```python
from build123d import *

# Parameters (mm, degrees)
ESQUISSE1_R             = 1.6
BOSS_EXTRU_1_DEPTH      = 3
BOSS_EXTRU_2_START      = 4
ESQUISSE2_R             = 2.734743529
ESQUISSE2_R_2           = 1.6
BOSS_EXTRU_2_DEPTH      = 4
ENL_V_MAT_EXTRU_1_DEPTH = 3


with BuildPart() as part:
    # Esquisse1 → Boss.-Extru.1 (new body)
    with BuildSketch(Plane(origin=(0, 0, 0), x_dir=(1, 0, 0), z_dir=(0, 1, 0))):
        with BuildLine():
            Line((-19, 3), (19, 3))
            add(Edge.make_bspline(
                [(19, 3), (20.68639149, 3.094620003), (23.315621509, 0.000753175), (20.682364624, -3.097569459), (19, -3)],
                knots=[0, 0, 0, 0, 0.499941737, 1, 1, 1, 1], degree=3))
            Line((19, -3), (-19, -3))
            add(Edge.make_bspline(
                [(-19, 3), (-20.661097815, 3.102497637), (-23.341647105, 0.00157467), (-20.655607875, -3.105760191), (-19, -3)],
                knots=[0, 0, 0, 0, 0.499995441, 1, 1, 1, 1], degree=3))
        make_face()
        with Locations(Location((-19, 0, 0), (0, 0, 270))):
            Circle(ESQUISSE1_R, mode=Mode.SUBTRACT)
        with Locations(Location((19, 0, 0), (0, 0, 90))):
            Circle(ESQUISSE1_R, mode=Mode.SUBTRACT)
    extrude(amount=BOSS_EXTRU_1_DEPTH)

    # Esquisse2 → Boss.-Extru.2 (add)
    with BuildSketch(Plane.XZ.offset(BOSS_EXTRU_2_START)):
        with Locations(Location((19, 0, 0), (0, 0, 270))):
            Circle(ESQUISSE2_R)
        with Locations(Location((19, 0, 0), (0, 0, 270))):
            Circle(ESQUISSE2_R_2, mode=Mode.SUBTRACT)
    extrude(amount=-BOSS_EXTRU_2_DEPTH)

    # Esquisse3 → Enlèv. mat.-Extru.1 (cut)
    with BuildSketch(Plane(origin=(0, 3, 0), x_dir=(1, 0, 0), z_dir=(0, 1, 0))):
        with BuildLine():
            Line((13.390376778, -1.25), (-13.390376778, -1.25))
            add(Edge.make_bspline(
                [(-13.390376778, -1.25), (-14.091002552, -1.290578927), (-15.1894504, 0.000117245), (-14.091603718, 1.290145329), (-13.390376778, 1.25)],
                knots=[0, 0, 0, 0, 0.500019288, 1, 1, 1, 1], degree=3))
            Line((-13.390376778, 1.25), (13.390376778, 1.25))
            add(Edge.make_bspline(
                [(13.390376778, -1.25), (14.084933338, -1.288382663), (15.205457343, -0.00659589), (14.065682357, 1.298551464), (13.390376778, 1.25)],
                knots=[0, 0, 0, 0, 0.500292138, 1, 1, 1, 1], degree=3))
        make_face()
    extrude(amount=-ENL_V_MAT_EXTRU_1_DEPTH, mode=Mode.SUBTRACT)


solid = part.part
```
The listing builds one solid part. Answer for the finished solid, in the listing's coordinates (mm). A direction names the side the tool comes from. Give positions to 0.01 mm unless a question says otherwise; leave off trailing zeros. Loops run counter-clockwise (first coordinate to the right, second up) from the corner with the lowest first, then second, coordinate; pieces in that order, holes last. Notation, with made-up numbers: (7.25, 15.5) - (15.25, 15.5) arc R12 ccw to (15.25, 33.5) - close; hole circle Ø7 at (66.25, 46). An arc over 180 degrees is marked (long way). Return JSON: item names as keys, results as strings. Group by question number.
1. Find section B-B (y = -2.25). Write down the section's boundary in (x, z), then the cut area to 3 significant figures.
2. Straight lines are drawn through the part: line 1 (X direction, y = 0.6, z = 0); line 2 (Z direction, x = -6, y = 2); line 3 (Z direction, x = 19, y = 2). For each, find the intervals that lie inside material, in ascending order. Write a range as [from, to].
3. Find section A-A (x = -8). Write down the section's boundary in (y, z).
4. Find section C-C (z = 0). State how many separate pieces and enclosed holes the cut face has, then the cut area to 3 significant figures.
5. Which of the six approach directions +Z, -Z, +X, -X, +Y, -Y give full straight-line access (tool end or side, diameter ignored) to faces 1 (the flat face through (0, 2, -1.25)), 2 (the flat face through (0.31, 3, -1.42))?
6. Determine the mould class of faces 3 (the cylindrical face through (21.71, -2.03, 0.36)), 4 (the flat face through (17, -4, 0)), 5 (the cylindrical face through (-17.414, 1.479, -0.208)) for opening direction X: pulls with the +X half, pulls with the -X half, needs draft (parallel to the pull), parting line crosses it, or undercut.
7. Given pin 1 Ø3 at (x, z) = (4, -0.5) entering from -Y; pin 2 Ø1 at (x, y) = (12, 0.5) entering from -Z; pin 3 Ø0.9 at (x, y) = (-6.5, 2) entering from +Z; pin 4 Ø3 at (x, z) = (-19, 0) entering from -Y, each flat-ended and moving along its own axis, determine where each tip first touches the part or whether it passes through.
Verdict:
{
 "1": {"outline": "circle Ø5.47 at (19, 0); hole circle Ø3.2 at (19, 0)", "area": "15.5 mm^2"},
 "2": {"line 1": "x = [-22, -20.6], [-17.4, -14.64], [14.64, 17.4], [20.6, 22]", "line 2": "z = [-3, -1.25], [1.25, 3]", "line 3": "z = [-3, -1.6], [1.6, 3]"},
 "3": {"outline": "(0, -3) - (3, -3) - (3, -1.25) - (0, -1.25) - close; (0, 1.25) - (3, 1.25) - (3, 3) - (0, 3) - close"},
 "4": {"separate pieces": "4", "enclosed holes": "0", "area": "34.0 mm^2"},
 "5": {"face 1": "+Y, -Y", "face 2": "+Z, -Z, +X, -X, +Y"},
 "6": {"face 3": "parting line crosses it", "face 4": "needs draft", "face 5": "undercut"},
 "7": {"pin 1": "stops at y = 0", "pin 2": "stops at z = -3", "pin 3": "stops at z = 3", "pin 4": "passes through"}
}
